from build123d import *

# Parameters (mm, degrees)
F1_DEPTH = 6.5
F2_W     = 13
F2_H     = 16
F2_W_2   = 9
F2_H_2   = 13
F3_DEPTH = 12
F4_R     = 4
F6_DEPTH = 33


with BuildPart() as f1:
    # F0 (on Right) → F1 (new body, symmetric)
    with BuildSketch(Plane.YZ):
        Polygon((5.2879960276, 8), (-38.7622783519, 8), (-38.7622783519, -8), (6.5257176757, -8), (41.2377216481, -12.1299560964), (40, 3.8700439036), align=None)
    extrude(amount=F1_DEPTH, both=True)

    # F2 (on face) → F3 (cut)
    with BuildSketch(Plane.XZ.offset(38.7622783519)):
        Rectangle(F2_W, F2_H)
        with Locations((0, 0.5)):
            Rectangle(F2_W_2, F2_H_2, mode=Mode.SUBTRACT)
    extrude(amount=-F3_DEPTH, mode=Mode.SUBTRACT)

    # F4
    f4_edges = [f1.edges().sort_by_distance(p)[0] for p in [
        (4.5, -32.762278, 7),
        (-4.5, -32.762278, 7),
        (4.5, -32.762278, -6),
        (-4.5, -32.762278, -6),
    ]]
    fillet(f4_edges, radius=F4_R)

    # F5 (on face) → F6 (cut)
    with BuildSketch(Plane.XZ.offset(26.7622783519)):
        with BuildLine():
            ThreePointArc((0, 8), (3.2708714327, 7.8149509816), (6.5, 7.2621655221))
            Line((6.5, 7.2621655221), (6.5, 8))
            Line((6.5, 8), (0, 8))
        make_face()
        with BuildLine():
            ThreePointArc((-6.5, 7.2621655221), (-3.2708714327, 7.8149509816), (0, 8))
            Line((0, 8), (-6.5, 8))
            Line((-6.5, 8), (-6.5, 7.2621655221))
        make_face()
        with BuildLine():
            Line((6.5, -8), (6.5, -7.2621655221))
            ThreePointArc((6.5, -7.2621655221), (3.2708714327, -7.8149509816), (0, -8))
            Line((0, -8), (6.5, -8))
        make_face()
        with BuildLine():
            Line((-6.5, -8), (0, -8))
            ThreePointArc((0, -8), (-3.2708714327, -7.8149509816), (-6.5, -7.2621655221))
            Line((-6.5, -7.2621655221), (-6.5, -8))
        make_face()
    extrude(amount=-F6_DEPTH, mode=Mode.SUBTRACT)


solid = f1.part
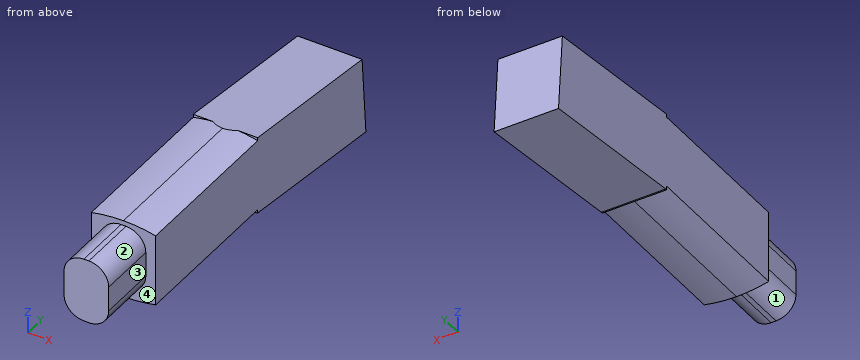
For this review, take the finished solid that the model builds, in its own axes (mm). Face numbers are marked on the shaded views. A direction names the side the tool comes from. Give positions to 0.01 mm unless a question says otherwise; leave off trailing zeros. Loops run counter-clockwise (first coordinate to the right, second up) from the corner with the lowest first, then second, coordinate; pieces in that order, holes last. Notation, with made-up numbers: (83.5, 71) - (94.5, 71) arc R31 ccw to (94.5, 97) - close; hole circle Ø2 at (69.25, -18.75). An arc over 180 degrees is marked (long way). Write each question's results on one line, items separated by ' | '.
(1) Take a section at B-B (x = 3.75). Give the boundary of the cut face in (y, z).
Conclusion:
outline: (-38.76, -4.33) - (-26.76, -4.33) - (-26.76, -7.76) - (6.24, -7.76) - (6.24, -8) - (6.53, -8) - (41.24, -12.13) - (40, 3.87) - (6.24, 7.89) - (6.24, 7.76) - (-26.76, 7.76) - (-26.76, 5.33) - (-38.76, 5.33) - close
(2) Take a section at C-C (z = 1). Give the boundary of the cut face in (x, y), then the cut area to 3 significant figures.
Conclusion:
outline: (-6.5, -26.76) - (-4.5, -26.76) - (-4.5, -38.76) - (4.5, -38.76) - (4.5, -26.76) - (6.5, -26.76) - (6.5, 40.22) - (-6.5, 40.22) - close | area: 979 mm^2
(3) For the marked faces 1, 2, 3 and 4, list the 3-axis set-ups (+Z, -Z, +X, -X, +Y, -Y) from which the entire face can be reached by the end or side of a thin tool; tool diameter is ignored.
Conclusion:
face 1: -Z, -X, -Y | face 2: +Z, +X, -Y | face 3: +Z, -Z, +X, -Y | face 4: -Y
(4) Take a section at A-A (y = -24). Give the boundary of the cut face in (x, z).
Conclusion:
outline: (-6.5, -7.26) arc R29 ccw to (6.5, -7.26) - (6.5, 7.26) arc R29 ccw to (-6.5, 7.26) - close
(5) Take a section at D-D (x = -5.5). Give the boundary of the cut face in (y, z).
Conclusion:
outline: (-26.76, -7.47) - (6.24, -7.47) - (6.24, -8) - (6.53, -8) - (41.24, -12.13) - (40, 3.87) - (6.24, 7.89) - (6.24, 7.47) - (-26.76, 7.47) - close
(6) For pin 1 Ø2 at (x, y) = (4.5, -7.5) entering from -Z; pin 2 Ø1 at (x, z) = (5, -8) entering from +Y; pin 3 Ø2 at (x, z) = (-1.5, 1.5) entering from +Y, all flat-tipped, find the tip position at first contact; note any pin that passes through.
Conclusion:
pin 1: z = -7.79 | pin 2: y = 40.96 | pin 3: y = 40.26
(7) For line 1 along X through (y, z) = (-28.5, 1.25); line 2 along Z through (x, y) = (-5.5, -13.5); line 3 along Y through (x, z) = (5.5, 1.75), list the stretches that pass through material, from the lowest coordinate up.
Conclusion:
line 1: -4.5 to 4.5 | line 2: -7.47 to 7.47 | line 3: -26.76 to 40.16
